Geometry: final body of the model. Coordinates: model frame, mm. Give positions to 0.01 mm unless a question says otherwise; leave off trailing zeros. Loops run counter-clockwise (first coordinate to the right, second up) from the corner with the lowest first, then second, coordinate; pieces in that order, holes last.
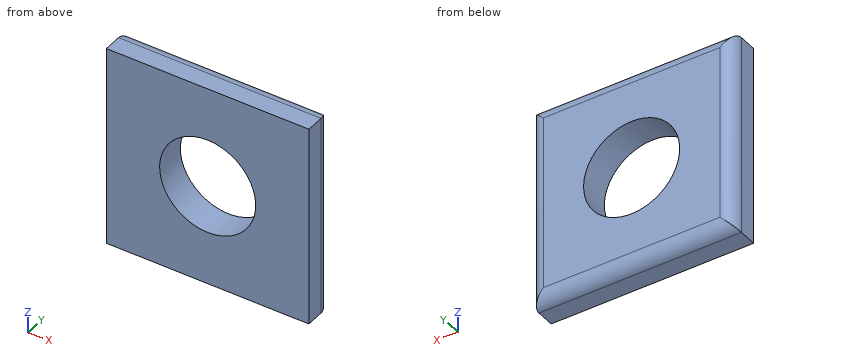
```python
from build123d import *

# Parameters (mm, degrees)
SKETCH_1_W          = 7.8
SKETCH_1_H          = 7.8
EXTRUDE_1_DEPTH     = 1.2
SKETCH_2_R          = 1.85
CUT_EXTRUDE_1_DEPTH = 1.2
FILLET_1_R          = 0.5


with BuildPart() as part:
    # 草图1 → 拉伸1 (new body)
    with BuildSketch(Plane(origin=(0, 0, 0), x_dir=(1, 0, 0), z_dir=(0, 1, 0))):
        Rectangle(SKETCH_1_W, SKETCH_1_H)
    extrude(amount=EXTRUDE_1_DEPTH)

    # 草图2 → 切除-拉伸1 (cut)
    with BuildSketch(Plane(origin=(0, 1.2, 0), x_dir=(-1, 0, 0), z_dir=(0, 1, 0))):
        with Locations(Location((0, 0, 0), (0, 0, 90))):
            Circle(SKETCH_2_R)
    extrude(amount=-CUT_EXTRUDE_1_DEPTH, mode=Mode.SUBTRACT)

    # 圆角1
    fillet_1_edges = [part.edges().sort_by_distance(p)[0] for p in [
        (3.9, 1.2, 0),
        (0, 1.2, -3.9),
        (-3.9, 1.2, 0),
        (0, 1.2, 3.9),
    ]]
    fillet(fillet_1_edges, radius=FILLET_1_R)


solid = part.part
```
Q1. Section query B-B, the plane z = 0. Return loops of the section in (x, y).
Q2. Section query D-D, the plane y = 0.15. Return loops of the section in (x, z), and give its area (3 significant figures).
Q3. Section query A-A, the plane x = 0. Return loops of the section in (y, z), and give its area (3 significant figures).
Q4. Pin query (flat end, axial travel): pin 1 Ø3.5 at (x, z) = (0, 0) entering from +Y; pin 2 Ø3 at (x, z) = (-2.5, -2) entering from -Y. Return the tip coordinate at first contact, or that it passes through.
Q5. Material intervals for probe 1 along X at (y, z) = (0.3, 0); probe 2 along Z at (x, y) = (-1, 0.95); probe 3 along X at (y, z) = (0.65, -0.75), sorted ascending.
Q6. Section query C-C, the plane y = 1.1. Return loops of the section in (x, z), and give its area (3 significant figures).
Resolved:
1. outline: (-3.9, 0) - (-1.85, 0) - (-1.85, 1.2) - (-3.4, 1.2) arc R0.5 ccw to (-3.9, 0.7) - close; (1.85, 0) - (3.9, 0) - (3.9, 0.7) arc R0.5 ccw to (3.4, 1.2) - (1.85, 1.2) - close
2. outline: (-3.9, -3.9) - (3.9, -3.9) - (3.9, 3.9) - (-3.9, 3.9) - close; hole circle Ø3.7 at (0, 0)
2. area: 50.1 mm2
3. outline: (0, -3.9) - (0.7, -3.9) arc R0.5 ccw to (1.2, -3.4) - (1.2, -1.85) - (0, -1.85) - close; (0, 1.85) - (1.2, 1.85) - (1.2, 3.4) arc R0.5 ccw to (0.7, 3.9) - (0, 3.9) - close
3. area: 4.81 mm2
4. pin 1: passes through
4. pin 2: stops at y = 0
5. probe 1: x = -3.9 to -1.85, 1.85 to 3.9
5. probe 2: z = -3.83 to -1.56, 1.56 to 3.83
5. probe 3: x = -3.9 to -1.69, 1.69 to 3.9
6. outline: (-3.7, -3.7) - (3.7, -3.7) - (3.7, 3.7) - (-3.7, 3.7) - close; hole circle Ø3.7 at (0, 0)
6. area: 44.0 mm2
